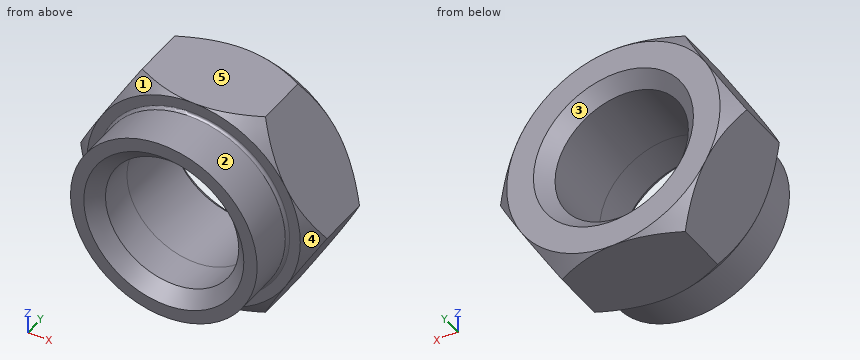
```python
from build123d import *

# Parameters (mm, degrees)
SZKIC1_R                    = 2.5
DODANIE_WYCI_GNI_CIE1_DEPTH = 3.2
SZKIC2_OUTSIDE_W            = 22.164
SZKIC2_OUTSIDE_H            = 20.926
SZKIC2_OUTSIDE_R            = 4
WYTNIJ_WYCI_GNI_CIE29_DEPTH = 4.2
WYTNIJ_WYCI_GNI_CIE29_TAPER = 45
SZKIC4_R                    = 3.5
SZKIC4_R_2                  = 2.5
DODANIE_WYCI_GNI_CIE2_DEPTH = 1.8
SZKIC5_OUTSIDE_W            = 33.878
SZKIC5_OUTSIDE_H            = 32.64
SZKIC5_OUTSIDE_R            = 4
WYTNIJ_WYCI_GNI_CIE30_DEPTH = 10
WYTNIJ_WYCI_GNI_CIE30_TAPER = 45
ZAOKR_GLENIE1_R             = 0.1
SFAZOWANIE1_SIZE            = 0.5


with BuildPart() as part:
    # Szkic1 → Dodanie-wyciągnięcie1 (new body)
    with BuildSketch(Plane(origin=(0, 0, 0), x_dir=(1, 0, 0), z_dir=(0, 1, 0))):
        Polygon((4.618802154, 0), (2.309401077, 4), (-2.309401077, 4), (-4.618802154, 0), (-2.309401077, -4), (2.309401077, -4), align=None)
        Circle(SZKIC1_R, mode=Mode.SUBTRACT)
    extrude(amount=DODANIE_WYCI_GNI_CIE1_DEPTH)

    # Szkic2 outside → Wytnij-wyciągnięcie29 (cut, through all)
    with BuildSketch(Plane(origin=(0, 3.2, 0), x_dir=(1, 0, 0), z_dir=(0, 1, 0))):
        Rectangle(SZKIC2_OUTSIDE_W, SZKIC2_OUTSIDE_H)
        Circle(SZKIC2_OUTSIDE_R, mode=Mode.SUBTRACT)
    extrude(amount=-WYTNIJ_WYCI_GNI_CIE29_DEPTH, taper=WYTNIJ_WYCI_GNI_CIE29_TAPER, mode=Mode.SUBTRACT)

    # Szkic4 → Dodanie-wyciągnięcie2 (add)
    with BuildSketch(Plane(origin=(0, 0, 0), x_dir=(-1, 0, 0), z_dir=(0, -1, 0))):
        Circle(SZKIC4_R)
        Circle(SZKIC4_R_2, mode=Mode.SUBTRACT)
    extrude(amount=DODANIE_WYCI_GNI_CIE2_DEPTH)

    # Szkic5 outside → Wytnij-wyciągnięcie30 (cut)
    with BuildSketch(Plane(origin=(0, 0, 0), x_dir=(-1, 0, 0), z_dir=(0, -1, 0))):
        Rectangle(SZKIC5_OUTSIDE_W, SZKIC5_OUTSIDE_H)
        Circle(SZKIC5_OUTSIDE_R, mode=Mode.SUBTRACT)
    extrude(amount=-WYTNIJ_WYCI_GNI_CIE30_DEPTH, taper=WYTNIJ_WYCI_GNI_CIE30_TAPER, mode=Mode.SUBTRACT)

    # Zaokrąglenie1
    zaokr_glenie1_edges = [part.edges().sort_by_distance(p)[0] for p in [
        (3.5, 0, 0),
    ]]
    fillet(zaokr_glenie1_edges, radius=ZAOKR_GLENIE1_R)

    # Sfazowanie1
    sfazowanie1_edges = [part.edges().sort_by_distance(p)[0] for p in [
        (-2.5, 3.2, 0),
        (2.5, -1.8, 0),
    ]]
    chamfer(sfazowanie1_edges, length=SFAZOWANIE1_SIZE)


solid = part.part
```
CAD build for the part. Positions are in the model's coordinates, mm. Face numbers are marked on the shaded views. A direction names the side the tool comes from. Give positions to 0.01 mm unless a question says otherwise; leave off trailing zeros. Write each loop counter-clockwise with the first axis right and the second up, starting at its lowest first coordinate (ties: lowest second). Pieces come first, ordered by that corner, then holes. Notation, with made-up numbers: (-2.75, 73) -> (14.25, 73) arc R27 cw to (14.25, 99) -> close; hole circle Ø9 at (57, 64). An arc over 180 degrees is marked (long way). Write each question's results on one line, items separated by ' | '.
1. Cut at A-A, the plane y = 1.5. Write the cut outline in (x, z), then the cut area to 3 significant figures.
Geometry check:
outline: (-4.62, 0) -> (-2.31, -4) -> (2.31, -4) -> (4.62, 0) -> (2.31, 4) -> (-2.31, 4) -> close; hole circle Ø5 at (0, 0) | area: 35.8 mm²
2. Drop a flat-ended pin along its axis: P1, Ø1, axis at y = -1, z = -2.5, coming from the +X side. Give the stop position or say it passes through.
Geometry check:
P1: x = 2.87
3. Wall check: probe 1 along Z at (x, y) = (0, -0.4); probe 2 along Z at (x, y) = (0, 1.15); probe 3 along X at (y, z) = (1.1, -0.5). Give the ranges that are in metal, low to high. Write a range as [from, to].
Geometry check:
probe 1: [-3.5, -2.5], [2.5, 3.5] | probe 2: [-4, -2.5], [2.5, 4] | probe 3: [-4.33, -2.45], [2.45, 4.33]
4. Two-plate mould, pull along X, no slides. Class the marked faces 3, 4 and 5: pulls with the +X half, pulls with the -X half, needs draft (parallel to the pull), parting line crosses it, or undercut.
Geometry check:
face 3: undercut | face 4: pulls with the +X half | face 5: needs draft
5. Cut at B-B, the plane y = 0.15. Write the cut outline in (x, z).
Geometry check:
outline: (-4.02, -1.04) -> (-2.91, -2.96) arc R4.15 ccw to (-1.11, -4) -> (1.11, -4) arc R4.15 ccw to (2.91, -2.96) -> (4.02, -1.04) arc R4.15 ccw to (4.02, 1.04) -> (2.91, 2.96) arc R4.15 ccw to (1.11, 4) -> (-1.11, 4) arc R4.15 ccw to (-2.91, 2.96) -> (-4.02, 1.04) arc R4.15 ccw to start; hole circle Ø5 at (0, 0)
6. Which spindle directions (+Z, -Z, +X, -X, +Y, -Y) get a long thin tool onto all of the face, cutting with end or side? Do the marked faces 1 and 2. Say none if no direction does.
Geometry check:
face 1: +Z, -X, -Y | face 2: -Y
